Geometry: see drawing. Coordinates: mm, zero at the bounding-box minimum. Give positions to 0.01 mm unless a question says otherwise; leave off trailing zeros. Loops run counter-clockwise (first coordinate to the right, second up) from the corner with the lowest first, then second, coordinate; pieces in that order, holes last. Notation, with made-up numbers: (-16.75, 88.5) -> (25.25, 88.5) arc R37 ccw to (25.25, 126.5) -> close; hole circle Ø11 at (22.5, 30.25). An arc over 180 degrees is marked (long way). One line per question, with ' | ' between items.
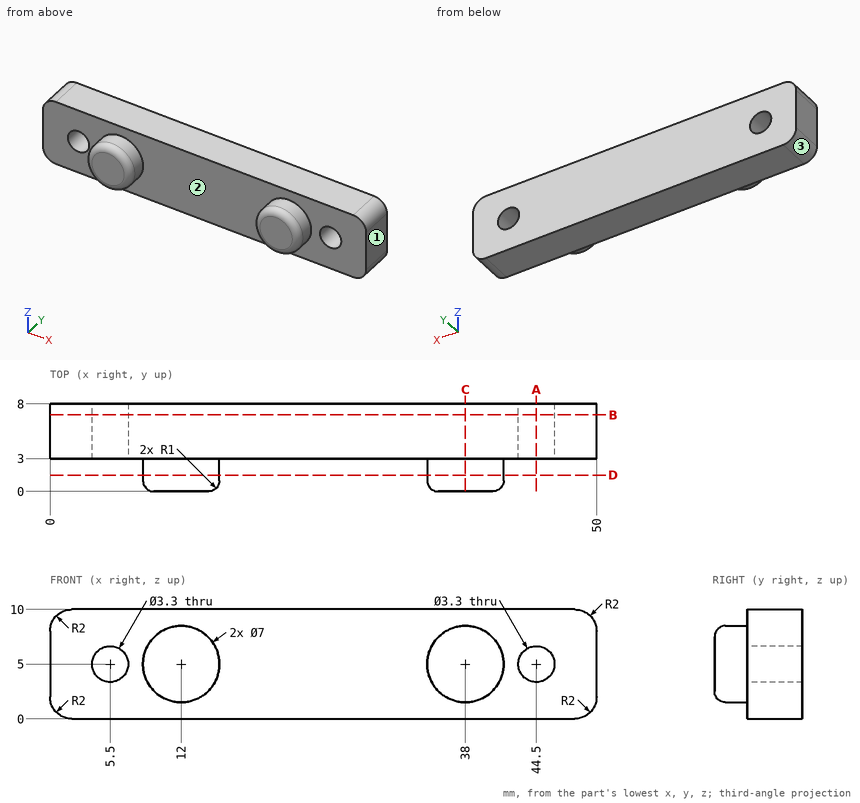
1. Ray query, line 1 along Z through (x, y) = (44.5, 6.3); line 2 along X through (y, z) = (6.5, 5.75); line 3 along X through (y, z) = (4.25, 4.5). Return the intervals inside material, ascending. Write a range as from..to.
Determined:
line 1: z = 0..3.35, 6.65..10 | line 2: x = 0..4.03, 6.97..43.03, 45.97..50 | line 3: x = 0..3.93, 7.07..42.93, 46.07..50
2. Pull-direction query (X, two-part tool) for the marked faces 1, 2 and 3; classes: pulls with the +X half, pulls with the -X half, needs draft (parallel to the pull), parting line crosses it, or undercut.
Determined:
face 1: pulls with the +X half | face 2: undercut | face 3: pulls with the -X half
3. Section query C-C (x = 38). Output: boundary loops of the cut face in (y, z).
Determined:
outline: (0, 2.5) arc R1 ccw to (1, 1.5) -> (3, 1.5) -> (3, 0) -> (8, 0) -> (8, 10) -> (3, 10) -> (3, 8.5) -> (1, 8.5) arc R1 ccw to (0, 7.5) -> close
4. Section query B-B (y = 7). Output: boundary loops of the cut face in (x, z).
Determined:
outline: (0, 2) arc R2 ccw to (2, 0) -> (48, 0) arc R2 ccw to (50, 2) -> (50, 8) arc R2 ccw to (48, 10) -> (2, 10) arc R2 ccw to (0, 8) -> close; hole circle Ø3.3 at (5.5, 5); hole circle Ø3.3 at (44.5, 5)
5. Pin query (flat end, axial travel): P1, Ø4, axis at x = 28, y = 2.5, coming from the -Z side; P2, Ø5, axis at x = 21.5, z = 3.5, coming from the -Y side. Return the tip coordinate at first contact, or that it passes through.
Determined:
P1: stops at z = 0 | P2: stops at y = 3
6. Section query A-A (x = 44.5). Output: boundary loops of the cut face in (y, z).
Determined:
outline: (3, 0) -> (8, 0) -> (8, 3.35) -> (3, 3.35) -> close; (3, 6.65) -> (8, 6.65) -> (8, 10) -> (3, 10) -> close
7. Section query D-D (y = 1.5). Output: boundary loops of the cut face in (x, z), then the cut area to 3 significant figures.
Determined:
outline: circle Ø7 at (12, 5); circle Ø7 at (38, 5) | area: 77.0 mm2
